from build123d import *

# Parameters (mm, degrees)
F0_W     = 47.9789283127
F0_H     = 24.23273772
F1_DEPTH = 75
F2_SIZE  = 5
F3_R     = 12.6691800878
F4_DEPTH = 24.23273772


with BuildPart() as f1:
    # F0 (on Right) → F1 (new body)
    with BuildSketch(Plane.YZ):
        with Locations((-44.6873651817, 47.6334765553)):
            Rectangle(F0_W, F0_H)
    extrude(amount=F1_DEPTH)

    # F2
    f2_edges = [f1.edges().sort_by_distance(p)[0] for p in [
        (37.5, -68.676829, 59.749845),
        (37.5, -20.697901, 59.749845),
        (75, -44.687365, 59.749845),
        (0, -44.687365, 59.749845),
    ]]
    chamfer(f2_edges, length=F2_SIZE)

    # F3 (on face) → F4 (cut, through all)
    with BuildSketch(Plane.XY.offset(59.7498454154)):
        with Locations((37.5, -44.6873651817)):
            Circle(F3_R)
    extrude(amount=-F4_DEPTH, mode=Mode.SUBTRACT)


solid = f1.part
Geometry: final body of the model. Coordinates: model frame, mm. Round coordinates to 2 decimals unless told otherwise and drop trailing zeros. Write each loop counter-clockwise with the first axis right and the second up, starting at its lowest first coordinate (ties: lowest second). Pieces come first, ordered by that corner, then holes. Notation, with made-up numbers: M 80,73.25 L 131,73.25 A22 ccw 131,106.25 Z; hole C 46.25,78.25 d1. An arc over 180 degrees is marked long. Write item = value, one per line.
Item 1: Section query A-A on x = 37.5. Return loops of the section in (y, z), then the cut area to 3 significant figures.
Findings:
outline = M -68.68,35.52 L -57.36,35.52 L -57.36,59.75 L -63.68,59.75 L -68.68,54.75 Z; M -32.02,35.52 L -20.7,35.52 L -20.7,54.75 L -25.7,59.75 L -32.02,59.75 Z
area = 524 mm^2
Item 2: Section query B-B on y = -50. Return loops of the section in (x, z), then the cut area to 3 significant figures.
Findings:
outline = M 0,35.52 L 26,35.52 L 26,59.75 L 5,59.75 L 0,54.75 Z; M 49,35.52 L 75,35.52 L 75,54.75 L 70,59.75 L 49,59.75 Z
area = 1,240 mm^2
Item 3: Section query C-C on z = 50.5. Return loops of the section in (x, y), then the cut area to 3 significant figures.
Findings:
outline = M 0,-68.68 L 75,-68.68 L 75,-20.7 L 0,-20.7 Z; hole C 37.5,-44.69 d25.34
area = 3,090 mm^2
Item 4: Section query D-D on x = 21.5. Return loops of the section in (y, z), then the cut area to 3 significant figures.
Findings:
outline = M -68.68,35.52 L -20.7,35.52 L -20.7,54.75 L -25.7,59.75 L -63.68,59.75 L -68.68,54.75 Z
area = 1,140 mm^2
Item 5: Pin query (flat end, axial travel): P1, Ø15, axis at x = 37.5, y = -44.69, coming from the -Z side. Return the tip coordinate at first contact, or that it passes through.
Findings:
P1 = through
Item 6: Material intervals for line 1 along Y through (x, z) = (37.5, 47.25); line 2 along X through (y, z) = (-41.5, 41.5); line 3 along X through (y, z) = (-52, 41.75), sorted ascending. Write a range as [from, to].
Findings:
line_1 = [-68.68, -57.36], [-32.02, -20.7]
line_2 = [0, 25.24], [49.76, 75]
line_3 = [0, 27.15], [47.85, 75]
Item 7: Pull-direction query (Y, two-part tool) for faces 1 (the face through (36.975, -66.142, 57.285)), 2 (the face through (36.97, -23.23, 57.28)), 3 (the face through (44.3, -34, 47.8)), 4 (the face through (37, -58, 59.75)); classes: pulls with the +Y half, pulls with the -Y half, needs draft (parallel to the pull), parting line crosses it, or undercut.
Findings:
face_1 = pulls with the -Y half
face_2 = pulls with the +Y half
face_3 = undercut
face_4 = needs draft
